Part model, mm, in its own coordinate system. A direction names the side the tool comes from. Give positions to 0.01 mm unless a question says otherwise; leave off trailing zeros. Write each loop counter-clockwise with the first axis right and the second up, starting at its lowest first coordinate (ties: lowest second). Pieces come first, ordered by that corner, then holes. Notation, with made-up numbers: M 22.25,43 L 80.25,43 A27 cw 80.25,82 Z; hole C -10,44.25 d6. An arc over 180 degrees is marked long. Use a Markdown table: item, result.
```python
from build123d import *

# Parameters (mm, degrees)
F0_W     = 127
F0_H     = 127
F1_DEPTH = 127
F2_R     = 12.7
F3_DEPTH = 6.35
F4_R     = 12.7
F5_DEPTH = 6.35
F6_DEPTH = 6.35
F7_R     = 12.7
F8_DEPTH = 6.35


with BuildPart() as f1:
    # F0 (on Top) → F1 (new body)
    with BuildSketch(Plane.XY):
        with Locations((0.547273, 11.179494)):
            Rectangle(F0_W, F0_H)
    extrude(amount=F1_DEPTH)

    # F2 (on face) → F3 (cut)
    with BuildSketch(Plane.XY.offset(127)):
        with Locations((0.547273, 11.179494)):
            Circle(F2_R)
    extrude(amount=-F3_DEPTH, mode=Mode.SUBTRACT)

    # F4 (on face) → F5 (join)
    with BuildSketch(Plane.YZ.offset(64.047273)):
        with Locations((46.731588, 99.052094)):
            Circle(F4_R)
        with Locations((-24.13532, 28.185186)):
            Circle(F4_R)
    extrude(amount=-F5_DEPTH)

    # F4 (on face) → F6 (cut)
    with BuildSketch(Plane.YZ.offset(64.047273)):
        with Locations((46.731588, 99.052094)):
            Circle(F4_R)
        with Locations((-24.13532, 28.185186)):
            Circle(F4_R)
    extrude(amount=-F6_DEPTH, mode=Mode.SUBTRACT)

    # F7 (on face) → F8 (cut)
    with BuildSketch(Plane.XZ.offset(52.320506)):
        with Locations((-40.727727, 104.775)):
            Circle(F7_R)
        with Locations((0, 64.047273)):
            Circle(F7_R)
        with Locations((41.822273, 22.225)):
            Circle(F7_R)
    extrude(amount=-F8_DEPTH, mode=Mode.SUBTRACT)


solid = f1.part
```
1. Tool access for faces 5 (the flat face through (0, -45.971, 64)), 6 (the flat face through (0, -52.321, 48)), 7 (the cylindrical face through (60.917, 45.078, 111.644)), 8 (the flat face through (-14, 12, 127)), 9 (the cylindrical face through (-9.53, 3.45, 123.87)): list every direction of +Z, -Z, +X, -X, +Y, -Y with a clear straight run to the whole face (end or side of a thin tool).
Findings below:
| item | result |
|---|---|
| face 5 | -Y |
| face 6 | +Z, -Z, +X, -X, -Y |
| face 7 | +X |
| face 8 | +Z, +X, -X, +Y, -Y |
| face 9 | +Z |
2. Drill centre lines: L1, parallel to Z at x = 0, y = -48; L2, parallel to Z at x = -6, y = 5. Where is each one in solid material? Low to high.
Findings below:
| item | result |
|---|---|
| L1 | 0 to 51.35, 76.75 to 127 |
| L2 | 0 to 120.65 |
3. Cut at B-B, the plane z = 20. Give the cut face in (x, y).
Findings below:
| item | result |
|---|---|
| outline | M -62.95,-52.32 L 29.32,-52.32 L 29.32,-45.97 L 54.33,-45.97 L 54.33,-52.32 L 64.05,-52.32 L 64.05,-33.85 L 57.7,-33.85 L 57.7,-14.42 L 64.05,-14.42 L 64.05,74.68 L -62.95,74.68 Z |
4. Drop flat-ended pins along their axis: P1, Ø12.5, axis at y = 45, z = 96.5, coming from the +X side; P2, Ø7.5, axis at x = -40.5, z = 110.5, coming from the -Y side. Give the stop position or say it passes through.
Findings below:
| item | result |
|---|---|
| P1 | x = 57.7 |
| P2 | y = -45.97 |
5. Two-plate mould, pull along X, no slides. Class faces 1 (the flat face through (0, 74.679, 63)), 2 (the cylindrical face through (39.069, -49.19, 9.827)), 3 (the flat face through (-62.953, 10, 63)), 4 (the flat face through (64.047, 10, 63)): released by +X, released by -X, zero draft, split by the parting line, or undercut.
Findings below:
| item | result |
|---|---|
| face 1 | zero draft |
| face 2 | undercut |
| face 3 | released by -X |
| face 4 | released by +X |
6. Cut at A-A, the plane x = -5. Give the cut face in (y, z).
Findings below:
| item | result |
|---|---|
| outline | M -52.32,0 L 74.68,0 L 74.68,127 L 22.6,127 L 22.6,120.65 L -0.24,120.65 L -0.24,127 L -52.32,127 L -52.32,75.72 L -45.97,75.72 L -45.97,52.37 L -52.32,52.37 Z |
